Model file for the job. Use its own axes, mm. Face numbers are marked on the shaded views. Give positions to 0.01 mm unless a question says otherwise; leave off trailing zeros. Loops run counter-clockwise (first coordinate to the right, second up) from the corner with the lowest first, then second, coordinate; pieces in that order, holes last. Notation, with made-up numbers: M 89,-32.75 L 109,-32.75 A26 cw 109,3.25 Z; hole C 73,-20 d3. An arc over 180 degrees is marked long. Answer in a Markdown table with one row per item.
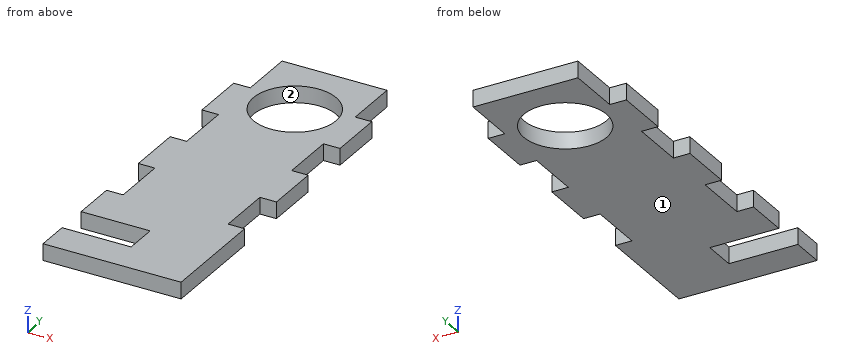
```python
from build123d import *

# Parameters (mm, degrees)
SKETCH1_W           = 25
SKETCH1_H           = 70
BOSS_EXTRUDE1_DEPTH = 3
SKETCH2_R           = 7.5
SKETCH2_W           = 3
SKETCH2_H           = 10
SKETCH2_W_2         = 12.5
SKETCH2_H_2         = 6
CUT_EXTRUDE1_DEPTH  = 3


with BuildPart() as part:
    # Sketch1 → Boss-Extrude1 (new body)
    with BuildSketch(Plane.XY):
        Rectangle(SKETCH1_W, SKETCH1_H)
    extrude(amount=BOSS_EXTRUDE1_DEPTH)

    # Sketch2 → Cut-Extrude1 (cut)
    with BuildSketch(Plane.XY.offset(3)):
        with Locations((0, 22.5)):
            Circle(SKETCH2_R)
        with Locations((-11, -10)):
            Rectangle(SKETCH2_W, SKETCH2_H)
        with Locations((11, 30)):
            Rectangle(SKETCH2_W, SKETCH2_H)
        with Locations((11, 10)):
            Rectangle(SKETCH2_W, SKETCH2_H)
        with Locations((11, -10)):
            Rectangle(SKETCH2_W, SKETCH2_H)
        with Locations((-11, 10)):
            Rectangle(SKETCH2_W, SKETCH2_H)
        with Locations((-11, 30)):
            Rectangle(SKETCH2_W, SKETCH2_H)
        with Locations((-6.25, -26)):
            Rectangle(SKETCH2_W_2, SKETCH2_H_2)
    extrude(amount=-CUT_EXTRUDE1_DEPTH, mode=Mode.SUBTRACT)


solid = part.part
```
Q1. Probe probe 1 along Y at (x, z) = (11, 2.3); probe 2 along Y at (x, z) = (1.5, 1.5); probe 3 along Y at (x, z) = (-8, 0.95). List the from-to ranges inside material, lowest first.
Reported:
| item | result |
|---|---|
| probe 1 | -35 to -15, -5 to 5, 15 to 25 |
| probe 2 | -35 to 15.15, 29.85 to 35 |
| probe 3 | -35 to -29, -23 to 35 |
Q2. Saw through at D-D (x = -8.75). Give the cut face in (y, z).
Reported:
| item | result |
|---|---|
| outline | M -35,0 L -29,0 L -29,3 L -35,3 Z; M -23,0 L 35,0 L 35,3 L -23,3 Z |
Q3. Drop flat-ended pins along their axis: pin 1 (0.9 mm diameter, centred on y = -24.5, z = 1.5, fed in from -X); pin 2 (0.9 mm diameter, centred on x = -11.5, z = 1.5, fed in from +Y); pin 3 (1.5 mm diameter, centred on y = 28.5, z = 2, fed in from +X). Give the stop position or say it passes through.
Reported:
| item | result |
|---|---|
| pin 1 | x = 0 |
| pin 2 | y = 25 |
| pin 3 | x = 9.5 |
Q4. Mould opens along Y. For the marked faces 1 and 2 say: released by +Y, released by -Y, zero draft, split by the parting line, or undercut.
Reported:
| item | result |
|---|---|
| face 1 | zero draft |
| face 2 | undercut |
Q5. Saw through at A-A (y = 22.5). Give the cut face in (x, z), and give its area (3 significant figures).
Reported:
| item | result |
|---|---|
| outline | M -12.5,0 L -7.5,0 L -7.5,3 L -12.5,3 Z; M 7.5,0 L 12.5,0 L 12.5,3 L 7.5,3 Z |
| area | 30.0 mm² |
Q6. Saw through at C-C (x = -6). Give the cut face in (y, z).
Reported:
| item | result |
|---|---|
| outline | M -35,0 L -29,0 L -29,3 L -35,3 Z; M -23,0 L 18,0 L 18,3 L -23,3 Z; M 27,0 L 35,0 L 35,3 L 27,3 Z |
